For this review, take the finished solid that the model builds, in its own axes (mm). A direction names the side the tool comes from. Give positions to 0.01 mm unless a question says otherwise; leave off trailing zeros. Write each loop counter-clockwise with the first axis right and the second up, starting at its lowest first coordinate (ties: lowest second). Pieces come first, ordered by that corner, then holes. Notation, with made-up numbers: (26.25, -32) -> (48.25, -32) arc R31 cw to (48.25, -7) -> close; hole circle Ø5 at (-39.5, 52.5). An arc over 180 degrees is marked (long way). Write item = value, one per line.
```python
from build123d import *

# Parameters (mm, degrees)
SKETCH1_W            = 80.01
SKETCH1_H            = 80.01
BOSS_EXTRUDE1_DEPTH  = 127
FILLET1_R            = 5.08
CUT_EXTRUDE1_DEPTH   = 140.031651253
MIRROR2_COPY_1_DEPTH = 140.031651253
MIRROR3_COPY_1_DEPTH = 140.031651253
MIRROR3_COPY_2_DEPTH = 140.031651253
MIRROR3_COPY_3_DEPTH = 140.031651253
FILLET2_R            = 1.27
CUT_EXTRUDE2_DEPTH   = 140.031651253
MIRROR5_COPY_1_DEPTH = 140.031651253
FILLET3_R            = 3.81
FILLET4_R            = 5.08


with BuildPart() as part:
    # Sketch1 → Boss-Extrude1 (new body)
    with BuildSketch(Plane.XY):
        Rectangle(SKETCH1_W, SKETCH1_H)
    extrude(amount=BOSS_EXTRUDE1_DEPTH)

    # Fillet1
    fillet1_edges = [part.edges().sort_by_distance(p)[0] for p in [
        (-40.005, 40.005, 63.5),
        (40.005, 40.005, 63.5),
        (40.005, -40.005, 63.5),
        (-40.005, -40.005, 63.5),
    ]]
    fillet(fillet1_edges, radius=FILLET1_R)

    # Sketch2 → Cut-Extrude1 (cut, through all)
    with BuildSketch(Plane.XY.offset(127)):
        Polygon((24.13, -40.005), (24.13, -35.433), (29.21, -35.433), (22.606, -28.829), (17.399, -28.829), (10.795, -35.433), (15.875, -35.433), (15.875, -40.005), align=None)
    cut_extrude1 = extrude(amount=-CUT_EXTRUDE1_DEPTH, mode=Mode.SUBTRACT)

    # Mirror1: Cut-Extrude1 across plane
    add(cut_extrude1.mirror(Plane(origin=(0, 0, 0), x_dir=(0, 0, 1), z_dir=(1, 0, 0))), mode=Mode.SUBTRACT)

    # Mirror2: Cut-Extrude1 across plane
    add(cut_extrude1.mirror(Plane.ZX), mode=Mode.SUBTRACT)

    # Mirror2 copy 1 sketch → Mirror2 copy 1 (cut, through all)
    with BuildSketch(Plane(origin=(0, 0, 127), x_dir=(-1, 0, 0), z_dir=(0, 0, 1))):
        Polygon((24.13, -40.005), (24.13, -35.433), (29.21, -35.433), (22.606, -28.829), (17.399, -28.829), (10.795, -35.433), (15.875, -35.433), (15.875, -40.005), align=None)
    extrude(amount=-MIRROR2_COPY_1_DEPTH, mode=Mode.SUBTRACT)

    # Mirror3: Cut-Extrude1 across plane
    add(cut_extrude1.mirror(Plane(origin=(0, 0, 0), x_dir=(0, 0, 1), z_dir=(0.7071067811865475, 0.7071067811865477, 0))), mode=Mode.SUBTRACT)

    # Mirror3 copy 1 sketch → Mirror3 copy 1 (cut, through all)
    with BuildSketch(Plane(origin=(0, 0, 127), x_dir=(0, 1, 0), z_dir=(0, 0, 1))):
        Polygon((24.13, -40.005), (24.13, -35.433), (29.21, -35.433), (22.606, -28.829), (17.399, -28.829), (10.795, -35.433), (15.875, -35.433), (15.875, -40.005), align=None)
    extrude(amount=-MIRROR3_COPY_1_DEPTH, mode=Mode.SUBTRACT)

    # Mirror3 copy 2 sketch → Mirror3 copy 2 (cut, through all)
    with BuildSketch(Plane(origin=(0, 0, 127), x_dir=(0, -1, 0), z_dir=(0, 0, 1))):
        Polygon((24.13, -40.005), (24.13, -35.433), (29.21, -35.433), (22.606, -28.829), (17.399, -28.829), (10.795, -35.433), (15.875, -35.433), (15.875, -40.005), align=None)
    extrude(amount=-MIRROR3_COPY_2_DEPTH, mode=Mode.SUBTRACT)

    # Mirror3 copy 3 sketch → Mirror3 copy 3 (cut, through all)
    with BuildSketch(Plane(origin=(0, 0, 127), x_dir=(0, 1, 0), z_dir=(0, 0, 1))):
        Polygon((24.13, 40.005), (24.13, 35.433), (29.21, 35.433), (22.606, 28.829), (17.399, 28.829), (10.795, 35.433), (15.875, 35.433), (15.875, 40.005), align=None)
    extrude(amount=-MIRROR3_COPY_3_DEPTH, mode=Mode.SUBTRACT)

    # Fillet2
    fillet2_edges = [part.edges().sort_by_distance(p)[0] for p in [
        (40.005, 24.13, 63.5),
        (40.005, 15.875, 63.5),
        (35.433, 15.875, 63.5),
        (35.433, 10.795, 63.5),
        (28.829, 17.399, 63.5),
        (28.829, 22.606, 63.5),
        (35.433, 29.21, 63.5),
        (35.433, 24.13, 63.5),
        (40.005, -15.875, 63.5),
        (40.005, -24.13, 63.5),
        (35.433, -24.13, 63.5),
        (35.433, -29.21, 63.5),
        (28.829, -22.606, 63.5),
        (28.829, -17.399, 63.5),
        (35.433, -10.795, 63.5),
        (35.433, -15.875, 63.5),
        (24.13, -40.005, 63.5),
        (15.875, -40.005, 63.5),
        (15.875, -35.433, 63.5),
        (10.795, -35.433, 63.5),
        (17.399, -28.829, 63.5),
        (22.606, -28.829, 63.5),
        (29.21, -35.433, 63.5),
        (24.13, -35.433, 63.5),
        (-15.875, -40.005, 63.5),
        (-24.13, -40.005, 63.5),
        (-24.13, -35.433, 63.5),
        (-29.21, -35.433, 63.5),
        (-22.606, -28.829, 63.5),
        (-17.399, -28.829, 63.5),
        (-10.795, -35.433, 63.5),
        (-15.875, -35.433, 63.5),
    ]]
    fillet(fillet2_edges, radius=FILLET2_R)

    # Sketch5 → Cut-Extrude2 (cut, through all)
    with BuildSketch(Plane.XY.offset(127)):
        Polygon((2.83202674, -32.893), (12.954, -22.77102674), (12.954, -12.954), (22.77102674, -12.954), (32.893, -2.83202674), (35.433, -2.83202674), (35.433, 0), (0, 0), (0, -35.433), (2.83202674, -35.433), align=None)
    cut_extrude2 = extrude(amount=-CUT_EXTRUDE2_DEPTH, mode=Mode.SUBTRACT)

    # Mirror4: Cut-Extrude2 across plane
    add(cut_extrude2.mirror(Plane.ZX), mode=Mode.SUBTRACT)

    # Mirror5: Cut-Extrude2 across plane
    add(cut_extrude2.mirror(Plane(origin=(0, 0, 0), x_dir=(0, 0, 1), z_dir=(1, 0, 0))), mode=Mode.SUBTRACT)

    # Mirror5 copy 1 sketch → Mirror5 copy 1 (cut, through all)
    with BuildSketch(Plane(origin=(0, 0, 127), x_dir=(-1, 0, 0), z_dir=(0, 0, 1))):
        Polygon((2.83202674, -32.893), (12.954, -22.77102674), (12.954, -12.954), (22.77102674, -12.954), (32.893, -2.83202674), (35.433, -2.83202674), (35.433, 0), (0, 0), (0, -35.433), (2.83202674, -35.433), align=None)
    extrude(amount=-MIRROR5_COPY_1_DEPTH, mode=Mode.SUBTRACT)

    # Fillet3
    fillet3_edges = [part.edges().sort_by_distance(p)[0] for p in [
        (12.954, -12.954, 63.5),
        (12.954, 12.954, 63.5),
        (-12.954, 12.954, 63.5),
        (-12.954, -12.954, 63.5),
    ]]
    fillet(fillet3_edges, radius=FILLET3_R)

    # Fillet4
    fillet4_edges = [part.edges().sort_by_distance(p)[0] for p in [
        (22.77102674, -12.954, 63.5),
        (12.954, -22.77102674, 63.5),
    ]]
    fillet(fillet4_edges, radius=FILLET4_R)


solid = part.part
```
(1) The part is to be moulded in two halves that separate along Y. For faces 4 (the face through (-38.556, -38.477, 64.389)), 5 (the face through (0, 40.005, 63)), 6 (the face through (20, 12.954, 64)), say which applies: released by +Y, released by -Y, zero draft, split by the parting line, or undercut.
Answers below:
face_4 = released by -Y
face_5 = released by +Y
face_6 = undercut
(2) To check wall thickness, follow probe 1 along Y at (x, z) = (-35.5, 117.5) (3 decimals); probe 2 along Y at (x, z) = (0, 54.5) (3 decimals); probe 3 along Y at (x, z) = (-32, 14.5) (3 decimals). State the ranges of each line that lie inside material, in increasing order.
Answers below:
probe_1 = -39.972 to -24.13, -15.875 to 15.875, 24.13 to 39.972
probe_2 = -40.005 to -35.433, 35.433 to 40.005
probe_3 = -40.005 to -25.777, -14.228 to -3.725, 3.725 to 14.228, 25.777 to 40.005
(3) Take a section at A-A (x = -20). Write out the cut boundary in (y, z), plus the area to 3 significant figures.
Answers below:
outline = (-28.83, 0) -> (-12.95, 0) -> (-12.95, 127) -> (-28.83, 127) -> close; (12.95, 0) -> (28.83, 0) -> (28.83, 127) -> (12.95, 127) -> close
area = 4,030 mm^2
(4) Tool access review of faces 1 (the face through (-38, 24.13, 64)), 2 (the face through (14.1, 14.04, 62.61)), 3 (the face through (28.829, 20, 64)): name each direction out of +Z, -Z, +X, -X, +Y, -Y from which nothing blocks a thin tool from reaching the whole face with its end or side.
Answers below:
face_1 = +Z, -Z, -X
face_2 = +Z, -Z
face_3 = +Z, -Z, +X
(5) For pin 1 (1.2 mm diameter, centred on y = 19.5, z = 56.5, fed in from +X); pin 2 (3.5 mm diameter, centred on y = 38, z = 42.5, fed in from -X); pin 3 (1.6 mm diameter, centred on y = -37.5, z = 75, fed in from -X); pin 4 (2 mm diameter, centred on x = 13.5, y = 13, fed in from +Z), all flat-tipped, find the tip position at first contact; note any pin that passes through.
Answers below:
pin_1 = 28.83
pin_2 = -39.83
pin_3 = -39.68
pin_4 = through
(6) Take a section at B-B (y = -8.5). Write out the cut boundary in (x, z) (3 decimals).
Answers below:
outline = (-40.005, 0) -> (-27.225, 0) -> (-27.225, 127) -> (-40.005, 127) -> close; (27.225, 0) -> (40.005, 0) -> (40.005, 127) -> (27.225, 127) -> close
